Check sheet for the drawn part. Datum: minimum x, y, z corner. Units: mm. A direction names the side the tool comes from. Coordinates: 2 decimals unless noted, no trailing zeros. Write each loop counter-clockwise with the first axis right and the second up, starting at its lowest first coordinate (ties: lowest second). Pieces come first, ordered by that corner, then holes. Notation, with made-up numbers: (41, 18) -> (79, 18) arc R21 ccw to (79, 27) -> close; hole circle Ø5 at (82, 52.25). An arc over 180 degrees is marked (long way). Answer in a Markdown table with one row per item.
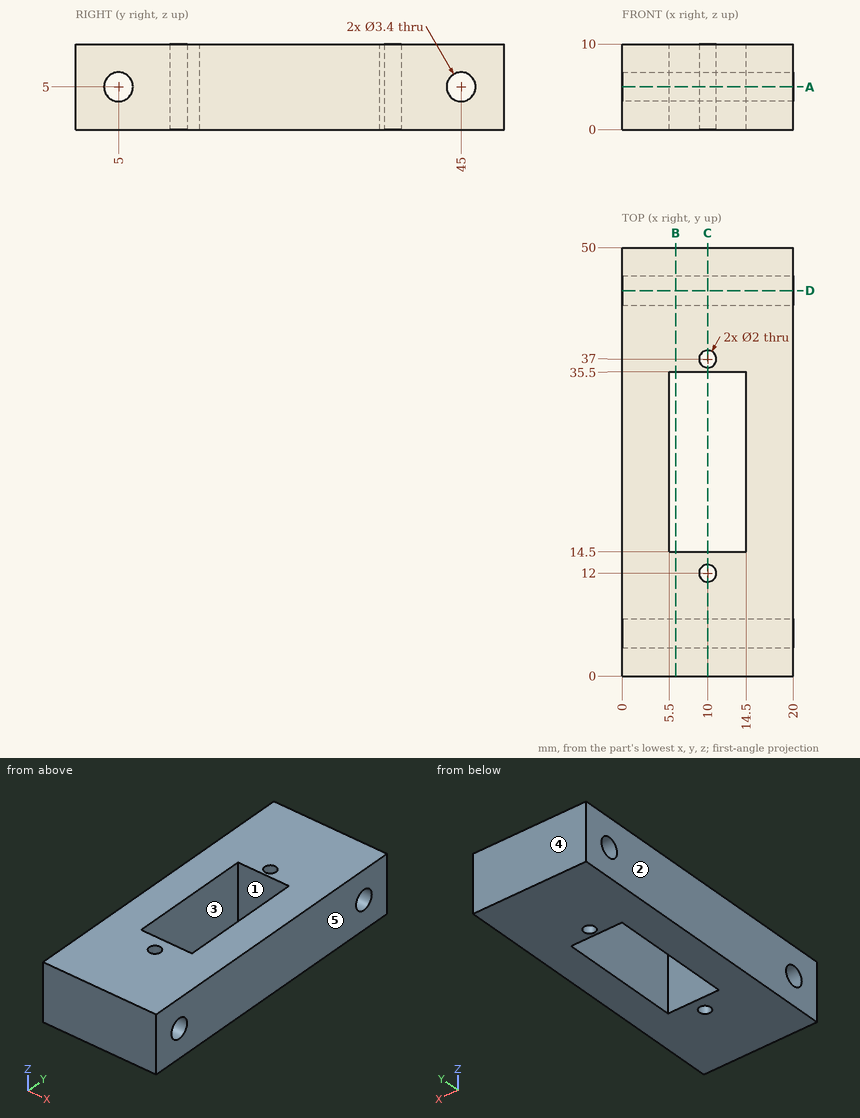
1. Sectioned sample at B-B, the plane x = 6.25. Record the cut outline in (y, z), and give its area (3 significant figures).
Findings below:
| item | result |
|---|---|
| outline | (0, 0) -> (14.5, 0) -> (14.5, 10) -> (0, 10) -> close; (35.5, 0) -> (50, 0) -> (50, 10) -> (35.5, 10) -> close; hole circle Ø3.4 at (5, 5); hole circle Ø3.4 at (45, 5) |
| area | 272 mm² |
2. Material ranges on probe 1 along Y at (x, z) = (10, 7); probe 2 along X at (y, z) = (18, 3.75); probe 3 along Y at (x, z) = (7.25, 2), recorded low to high. Write a range as from..to.
Findings below:
| item | result |
|---|---|
| probe 1 | y = 0..11, 13..14.5, 35.5..36, 38..50 |
| probe 2 | x = 0..5.5, 14.5..20 |
| probe 3 | y = 0..14.5, 35.5..50 |
3. Sectioned sample at A-A, the plane z = 5. Record the cut outline in (x, y), and give its area (3 significant figures).
Findings below:
| item | result |
|---|---|
| outline | (0, 0) -> (20, 0) -> (20, 3.3) -> (0, 3.3) -> close; (0, 6.7) -> (20, 6.7) -> (20, 43.3) -> (0, 43.3) -> close; (0, 46.7) -> (20, 46.7) -> (20, 50) -> (0, 50) -> close; hole (5.5, 14.5) -> (14.5, 14.5) -> (14.5, 35.5) -> (5.5, 35.5) -> close; hole circle Ø2 at (10, 12); hole circle Ø2 at (10, 37) |
| area | 669 mm² |
4. Access from +Z, -Z, +X, -X, +Y, -Y to the whole of each face (thin tool, end or side, straight path). Record for the marked faces 1 and 2.
Findings below:
| item | result |
|---|---|
| face 1 | +Z, -Z |
| face 2 | +Z, -Z, -X, +Y, -Y |
5. Go/stop test with a flat-tipped pin: pin 1 (3 mm diameter, centred on y = 45, z = 5, fed in from -X). Record where the tip stops, or that it passes through.
Findings below:
| item | result |
|---|---|
| pin 1 | passes through |
6. Sectioned sample at D-D, the plane y = 45. Record the cut outline in (x, z).
Findings below:
| item | result |
|---|---|
| outline | (0, 0) -> (20, 0) -> (20, 3.3) -> (0, 3.3) -> close; (0, 6.7) -> (20, 6.7) -> (20, 10) -> (0, 10) -> close |
7. Sectioned sample at C-C, the plane x = 10. Record the cut outline in (y, z), and give its area (3 significant figures).
Findings below:
| item | result |
|---|---|
| outline | (0, 0) -> (11, 0) -> (11, 10) -> (0, 10) -> close; (13, 0) -> (14.5, 0) -> (14.5, 10) -> (13, 10) -> close; (35.5, 0) -> (36, 0) -> (36, 10) -> (35.5, 10) -> close; (38, 0) -> (50, 0) -> (50, 10) -> (38, 10) -> close; hole circle Ø3.4 at (5, 5); hole circle Ø3.4 at (45, 5) |
| area | 232 mm² |
8. Release check for a two-part mould opening along X. For the marked faces 3, 4 and 5 record: released by +X, released by -X, zero draft, split by the parting line, or undercut.
Findings below:
| item | result |
|---|---|
| face 3 | undercut |
| face 4 | zero draft |
| face 5 | released by +X |
